```python
from build123d import *

# Parameters (mm, degrees)
BOSS_EXTRUDE1_DEPTH     = 23
SKETCH2_W               = 18
SKETCH2_H               = 18
BOSS_EXTRUDE2_DEPTH     = 20
CUT_EXTRUDE1_DEPTH      = 76.193084788
CUT_EXTRUDE1_DEPTH_BACK = 76.193084788
SKETCH3_R               = 4
SKETCH4_R               = 20
BOSS_EXTRUDE3_DEPTH     = 95
SKETCH5_R               = 10
BOSS_EXTRUDE4_DEPTH     = 150


with BuildPart() as part:
    # Sketch1 → Boss-Extrude1 (new body)
    with BuildSketch(Plane(origin=(0, 0, 0), x_dir=(1, 0, 0), z_dir=(0, 1, 0))):
        with BuildLine():
            Line((-21, -24), (21, -24))
            Line((21, -24), (21, 37))
            ThreePointArc((21, 37), (0, 58), (-21, 37))
            Line((-21, 37), (-21, -24))
        make_face()
    extrude(amount=-BOSS_EXTRUDE1_DEPTH)

    # Sketch2 → Boss-Extrude2 (add)
    with BuildSketch(Plane.XZ.offset(23)):
        Rectangle(SKETCH2_W, SKETCH2_H)
    extrude(amount=BOSS_EXTRUDE2_DEPTH)

    # Sketch3 → Cut-Extrude1 (cut, two sides: drawn at the far end of the back side and taken through both)
    with BuildSketch(Plane(origin=(0, 0, 0), x_dir=(0, 0, -1), z_dir=(1, 0, 0)).offset(-CUT_EXTRUDE1_DEPTH_BACK)):
        with Locations((0, -35)):
            Circle(SKETCH3_R)
    extrude(amount=CUT_EXTRUDE1_DEPTH + CUT_EXTRUDE1_DEPTH_BACK, mode=Mode.SUBTRACT)

    # Sketch4 → Boss-Extrude3 (add)
    with BuildSketch(Plane.XZ.offset(23)):
        with Locations(Location((0, -37, 0), (0, 0, 270))):
            Circle(SKETCH4_R)
    extrude(amount=-BOSS_EXTRUDE3_DEPTH)

    # Sketch5 → Boss-Extrude4 (add)
    with BuildSketch(Plane(origin=(0, 0, 0), x_dir=(1, 0, 0), z_dir=(0, 1, 0))):
        with BuildLine():
            Line((-15.25, 0), (-15.25, -20.75))
            Line((-15.25, -20.75), (15.25, -20.75))
            Line((15.25, -20.75), (15.25, 0))
            ThreePointArc((15.25, 0), (0, 15.25), (-15.25, 0))
        make_face()
        with Locations(Location((0, 0, 0), (0, 0, 270))):
            Circle(SKETCH5_R, mode=Mode.SUBTRACT)
    extrude(amount=BOSS_EXTRUDE4_DEPTH)


solid = part.part
```
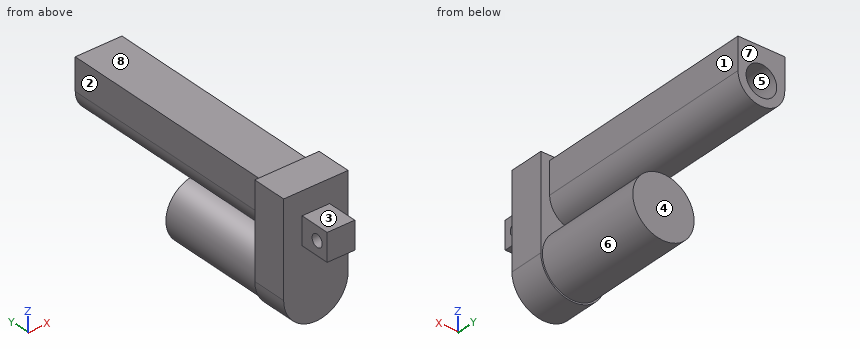
Check sheet for the modelled part. Datum: model origin and axes. Units: mm. Face numbers are marked on the shaded views. A direction names the side the tool comes from. Coordinates: 2 decimals unless noted, no trailing zeros. Order: outer loops, then holes, each group sorted by start corner. A loop starts at its lowest first (then second) coordinate and runs counter-clockwise, first axis right, second up. Notation, with made-up numbers: (-31, 82.5) -> (-13, 82.5) arc R29 ccw to (-13, 104.5) -> close; hole circle Ø9 at (-28, -2). An arc over 180 degrees is marked (long way). Write item = value, one per line. Start each with the question number.
1) Go/stop test with flat-tipped pins: P1, Ø10, axis at y = 92.5, z = 1.5, coming from the +X side; P2, Ø12, axis at x = -2, z = -31, coming from the -Y side; P3, Ø5.5, axis at y = -28, z = 2, coming from the -X side; P4, Ø5, axis at y = -35, z = 0, coming from the +X side. Record where each tip stops, or that it passes through.
2) Mould release check, pull along Z, two halves, no side actions. Record for the marked faces 6, 7 and 8: +Z half, -Z half, draft (parallel to the pull), parting line (faces both ways), or undercut.
3) Cross-section at D-D (x = -18). Enter the section's corners in (y, z).
4) Cross-section at B-B (x = 0). Enter the section's corners in (y, z), then the cut area to 3 significant figures.
5) Cross-section at A-A (y = 101.5). Enter the section's corners in (x, z).
6) Cross-section at C-C (z = 16.5). Enter the section's corners in (x, y), then the cut area to 3 significant figures.
7) Access from +Z, -Z, +X, -X, +Y, -Y to the whole of each face (thin tool, end or side, straight path). Record for the marked faces 1, 2, 3, 4 and 5.
8) Material ranges on L1, parallel to X at y = 72, z = 0; L2, parallel to Y at x = 2, z = 0; L3, parallel to Z at x = -3, y = -35, recorded low to high.
Ans:
q1.P1 = 15.25
q1.P2 = -23
q1.P3 = -9
q1.P4 = through
q2.face_6 = undercut
q2.face_7 = draft
q2.face_8 = +Z half
q3.outline = (-23, -47.82) -> (0, -47.82) -> (0, -45.72) -> (72, -45.72) -> (72, -28.28) -> (0, -28.28) -> (0, 24) -> (-23, 24) -> close
q4.outline = (-43, -9) -> (-23, -9) -> (-23, -58) -> (0, -58) -> (0, -57) -> (72, -57) -> (72, -17) -> (0, -17) -> (0, -15.25) -> (150, -15.25) -> (150, -10) -> (0, -10) -> (0, 10) -> (150, 10) -> (150, 20.75) -> (0, 20.75) -> (0, 24) -> (-23, 24) -> (-23, 9) -> (-43, 9) -> close; hole circle Ø8 at (-35, 0)
q4.area = 7,480 mm²
q5.outline = (-15.25, 0) arc R15.25 ccw to (15.25, 0) -> (15.25, 20.75) -> (-15.25, 20.75) -> close; hole circle Ø20 at (0, 0)
q6.outline = (-21, -23) -> (21, -23) -> (21, 0) -> (15.25, 0) -> (15.25, 150) -> (-15.25, 150) -> (-15.25, 0) -> (-21, 0) -> close
q6.area = 5,540 mm²
q7.face_1 = +Z, +X, +Y
q7.face_2 = +Z, -X, +Y
q7.face_3 = +Z, +X, -X, -Y
q7.face_4 = -Z, +X, -X, +Y
q7.face_5 = +Y
q8.L1 = -15.25 to -10, 10 to 15.25
q8.L2 = -43 to -39, -31 to 0
q8.L3 = -9 to -4, 4 to 9
